Check sheet for the drawn part. Datum: minimum x, y, z corner. Units: mm. Round coordinates to 2 decimals unless told otherwise and drop trailing zeros. Order: outer loops, then holes, each group sorted by start corner. A loop starts at its lowest first (then second) coordinate and runs counter-clockwise, first axis right, second up. Notation, with made-up numbers: (-10.5, 15) -> (-3.5, 15) arc R17 cw to (-3.5, 37) -> close; hole circle Ø7 at (81.25, 61.5). An arc over 180 degrees is marked (long way). Write item = value, one per line. Start each with the question number.
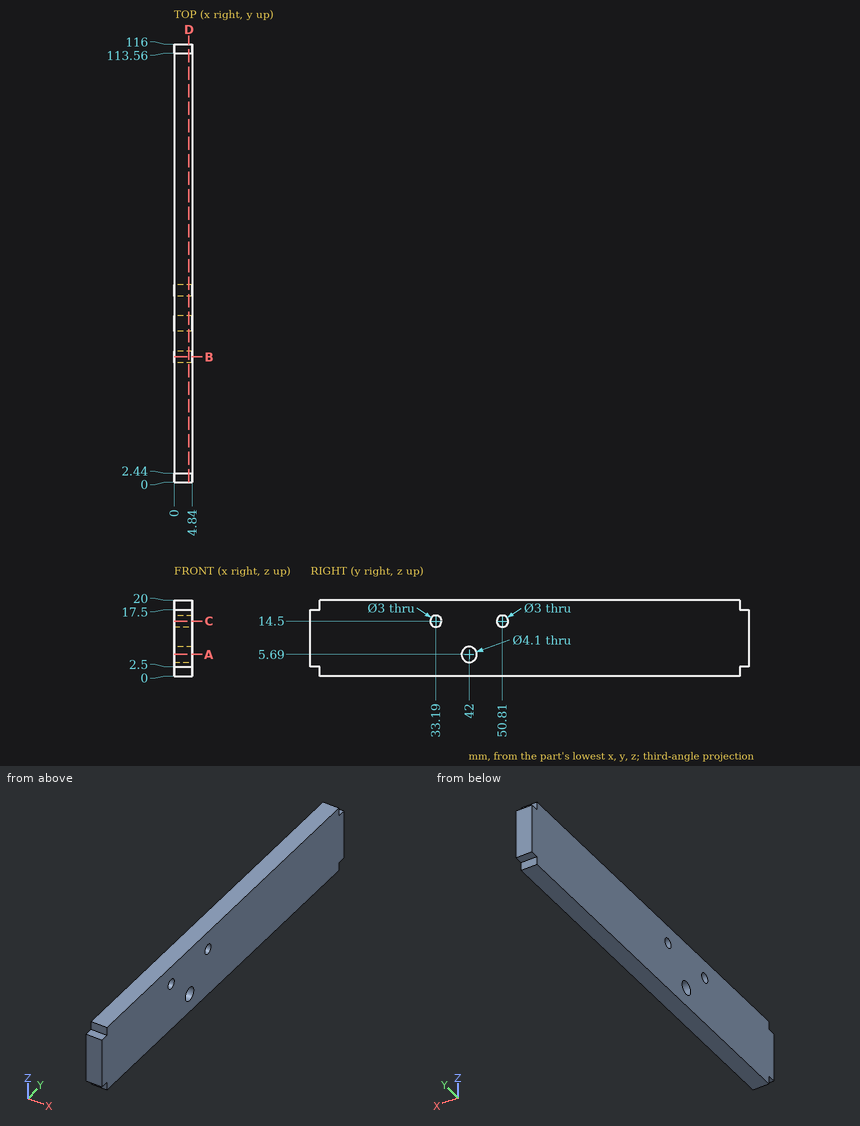
(1) Cross-section at D-D (x = 3.9). Enter the section's corners in (y, z), and give its area (3 significant figures).
(2) Cross-section at B-B (y = 33.19). Enter the section's corners in (x, z).
(3) Cross-section at C-C (z = 14.5). Enter the section's corners in (x, y), and give its area (3 significant figures).
(4) Depth check by flat-ended pin: pin 1 (2 mm diameter, centred on x = 3.5, y = 2, fed in from +Z); pin 2 (1.2 mm diameter, centred on x = 3.5, z = 18.5, fed in from -Y); pin 3 (2.5 mm diameter, centred on x = 2, y = 115.5, fed in from -Z); pin 4 (2 mm diameter, centred on x = 3, z = 1, fed in from +Y). Enter the tip coordinate at first touch or a pass-through.
(5) Cross-section at A-A (z = 5.69). Enter the section's corners in (x, y).
(6) Scan lines: line 1 along Y through (x, z) = (3.1, 14.5); line 2 along Y through (x, z) = (2.85, 5.69); line 3 along Y through (x, z) = (4.3, 1.5). Record each from-to range of solid material in increasing order. Write a range as from..to.
Outcome:
q1.outline = (0, 2.5) -> (2.44, 2.5) -> (2.44, 0) -> (113.56, 0) -> (113.56, 2.5) -> (116, 2.5) -> (116, 17.5) -> (113.56, 17.5) -> (113.56, 20) -> (2.44, 20) -> (2.44, 17.5) -> (0, 17.5) -> close; hole circle Ø3 at (33.19, 14.5); hole circle Ø4.1 at (42, 5.69); hole circle Ø3 at (50.81, 14.5)
q1.area = 2,270 mm^2
q2.outline = (0, 0) -> (4.84, 0) -> (4.84, 13) -> (0, 13) -> close; (0, 16) -> (4.84, 16) -> (4.84, 20) -> (0, 20) -> close
q3.outline = (0, 0) -> (4.84, 0) -> (4.84, 31.69) -> (0, 31.69) -> close; (0, 34.69) -> (4.84, 34.69) -> (4.84, 49.31) -> (0, 49.31) -> close; (0, 52.31) -> (4.84, 52.31) -> (4.84, 116) -> (0, 116) -> close
q3.area = 532 mm^2
q4.pin_1 = 20
q4.pin_2 = 2.44
q4.pin_3 = 2.5
q4.pin_4 = 113.56
q5.outline = (0, 0) -> (4.84, 0) -> (4.84, 39.95) -> (0, 39.95) -> close; (0, 44.05) -> (4.84, 44.05) -> (4.84, 116) -> (0, 116) -> close
q6.line_1 = 0..31.69, 34.69..49.31, 52.31..116
q6.line_2 = 0..39.95, 44.05..116
q6.line_3 = 2.44..113.56
